Autodesk Inventor part; units mm, degrees
ref_plane "YZ Plane" through (0, 0, 0) normal (1, 0, 0) x (0, 1, 0)
ref_plane "XZ Plane" through (0, 0, 0) normal (0, 1, 0) x (-1, 0, 0)
ref_plane "XY Plane" through (0, 0, 0) normal (0, 0, 1) x (1, 0, 0)
sketch "Sketch1" plane through (0, 0, 0) normal (0, 0, 1) x (1, 0, 0)
  line L0 (-12.1708, 16.0073) -> (13.2292, 16.0073)
  line L1 (13.2292, 16.0073) -> (13.2292, -34.7927)
  line L2 (13.2292, -34.7927) -> (-12.1708, -34.7927)
  line L3 (-12.1708, -34.7927) -> (-12.1708, 16.0073)
  line L4 (11.9592, 14.7373) -> (-10.9008, 14.7373)
  line L5 (-10.9008, 14.7373) -> (-10.9008, -33.5227)
  line L6 (-10.9008, -33.5227) -> (11.9592, -33.5227)
  line L7 (11.9592, -33.5227) -> (11.9592, 14.7373)
  point P0 (0, 0)
  dimension "d0" = 25.4
  dimension "d1" = 50.8
  dimension "d2" = 1.27
extrude "Extrusion1" add sketch "Sketch1" along normal blind 228.6
sketch "Sketch2" plane through (-12.1708, 16.0073, 0) normal (0, 1, 0) x (1, 0, 0)
  circle A0 centre (12.7, -12.7) radius 1.7272
  line L0 (25.4, 0) -> (0, 0)
  line L1 (0, 0) -> (0, -228.6)
  point P0 (12.1708, 0)
  dimension "d5" = 3.4544
  dimension "d6" = 12.7
  dimension "d7" = 12.7
extrude "Extrusion2" cut sketch "Sketch2" against normal through all
pattern_linear "Rectangular Pattern1" count 71 spacing 25.4 along (0, 0, 1) of "Extrusion2"
sketch "Sketch4" plane through (13.2292, -34.7927, 0) normal (1, 0, 0) x (0, 0, -1)
  circle A0 centre (-82.55, 25.4) radius 14.2875
  line L0 (0, 50.8) -> (-228.6, 50.8)
  line L1 (0, 0) -> (0, 50.8)
  line L2 (0, 50.8) -> (-228.6, 50.8)
  line L3 (-228.6, 0) -> (-228.6, 50.8)
  line L4 (0, 0) -> (-228.6, 0)
  circle A1 centre (-184.15, 25.4) radius 14.2875
  point P0 (0, 34.7927)
  point P1 (0, 25.4)
  dimension "d31" = 28.575
  dimension "d34" = 28.575
  dimension "d35" = 44.45
  dimension "d36" = 25.4
  dimension "d39" = 101.6
extrude "Extrusion4" cut sketch "Sketch4" against normal blind 25.4 contours A0 | A1
equation "\"d10\" = d14"
equation "\"d13\" = 711.2"
equation "\"d14\" = d13"
properties part number "VersaFrame_VelcRail2"
Work out the finished part from the listing and answer in its coordinate system (mm). A direction names the side the tool comes from. Give positions to 0.01 mm unless a question says otherwise; leave off trailing zeros. Order: outer loops, then holes, each group sorted by start corner. A loop starts at its lowest first (then second) coordinate and runs counter-clockwise, first axis right, second up. Notation, with made-up numbers: M 58,-28 L 117,-28 A22 ccw 117,-9 Z; hole C 81.25,-34 d7. An arc over 180 degrees is marked long. Return JSON: item names as keys, results as strings.
Q1. Find the intervals of material crossed by line 1 along Y through (x, z) = (8, 158); line 2 along X through (y, z) = (-31, 26.5); line 3 along X through (y, z) = (15.2, 63.5), in increasing order. Write a range as [from, to].
Answer below:
{"line 1": "y = [-34.79, -33.52], [14.74, 16.01]", "line 2": "x = [-12.17, -10.9], [11.96, 13.23]", "line 3": "x = [-12.17, -1.2], [2.26, 13.23]"}
Q2. The mould has two halves that part along X. Classify faces 3 (the face through (-2, -33.523, 113)), 4 (the face through (-12.171, -10, 113)), 5 (the face through (-11.527, -5.101, 68.922)), 6 (the face through (11.959, -10, 113)): pulls with the +X half, pulls with the -X half, needs draft (parallel to the pull), parting line crosses it, or undercut.
Answer below:
{"face 3": "undercut", "face 4": "pulls with the -X half", "face 5": "needs draft", "face 6": "undercut"}
Q3. Which of the six approach directions +Z, -Z, +X, -X, +Y, -Y give full straight-line access (tool end or side, diameter ignored) to faces 1 (the face through (-10.901, -9, 113)), 2 (the face through (12.603, -5.101, 68.922))?
Answer below:
{"face 1": "+Z, -Z", "face 2": "+X, -X"}
Q4. Find section D-D, the plane z = 179. Write down the section's boundary in (x, y), and give its area (3 significant figures).
Answer below:
{"outline": "M -12.17,-34.79 L 13.23,-34.79 L 13.23,-22.72 L 11.96,-22.72 L 11.96,-33.52 L -10.9,-33.52 L -10.9,-22.72 L -12.17,-22.72 Z; M -12.17,3.93 L -10.9,3.93 L -10.9,14.74 L 11.96,14.74 L 11.96,3.93 L 13.23,3.93 L 13.23,16.01 L -12.17,16.01 Z", "area": "119 mm^2"}
Q5. This flat-tipped pin is pushed along its axis until it touches: pin 1 (3 mm diameter, centred on x = -0.5, z = 164.5, fed in from -Y). Where does it stop, or does it pass through?
Answer below:
{"pin 1": "stops at y = -34.79"}
Q6. Find section B-B, the plane x = 7. Write down the section's boundary in (y, z).
Answer below:
{"outline": "M -34.79,0 L -33.52,0 L -33.52,228.6 L -34.79,228.6 Z; M 14.74,0 L 16.01,0 L 16.01,228.6 L 14.74,228.6 Z"}
Q7. Find section A-A, the plane y = -27.5. Write down the section's boundary in (x, z), and give its area (3 significant figures).
Answer below:
{"outline": "M -12.17,0 L -10.9,0 L -10.9,228.6 L -12.17,228.6 Z; M 11.96,0 L 13.23,0 L 13.23,228.6 L 11.96,228.6 Z", "area": "581 mm^2"}
Q8. Find section C-C, the plane y = -18. Write down the section's boundary in (x, z).
Answer below:
{"outline": "M -12.17,0 L -10.9,0 L -10.9,71.15 L -12.17,71.15 Z; M -12.17,93.95 L -10.9,93.95 L -10.9,172.75 L -12.17,172.75 Z; M -12.17,195.55 L -10.9,195.55 L -10.9,228.6 L -12.17,228.6 Z; M 11.96,0 L 13.23,0 L 13.23,71.15 L 11.96,71.15 Z; M 11.96,93.95 L 13.23,93.95 L 13.23,172.75 L 11.96,172.75 Z; M 11.96,195.55 L 13.23,195.55 L 13.23,228.6 L 11.96,228.6 Z"}
